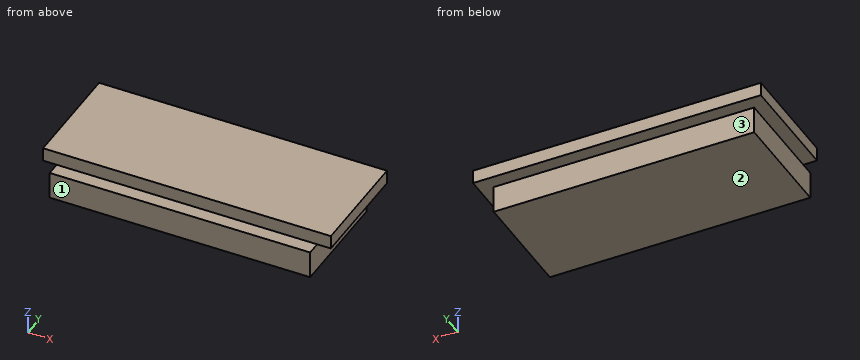
Autodesk Fusion 360 part; units mm, degrees
sketch "Sketch1" plane through (0, 0, 0) normal (0, 0, 1) x (1, 0, 0)
  line L0 (9.5, 4) -> (-9.5, 4)
  line L1 (-9.5, 4) -> (-9.5, -4)
  line L2 (-9.5, -4) -> (9.5, -4)
  line L3 (9.5, -4) -> (9.5, 4)
  line L4 (9.5, 4) -> (-9.5, -4) construction
  line L5 (-9.5, 4) -> (9.5, -4) construction
  dimension "d1" = 19
  dimension "d2" = 8
extrude "Extrude1" add sketch "Sketch1" along normal blind 2
sketch "Sketch2" plane through (0, 0, 2) normal (0, 0, 1) x (-1, 0, 0)
  line L0 (-9.5, 4) -> (-9.5, -4)
  line L1 (-9.5, -4) -> (9.5, -4)
  line L2 (9.5, -4) -> (9.5, 4)
  line L3 (9.5, 4) -> (-9.5, 4)
  line L4 (0, 4) -> (0, 3)
  line L5 (0, 3) -> (0, -5)
  line L6 (-10.5, -5) -> (10.5, -5)
  line L7 (10.5, -5) -> (10.5, 3)
  line L8 (10.5, 3) -> (-10.5, 3)
  line L9 (-10.5, 3) -> (-10.5, -5)
  line L10 (-10.5, -5) -> (10.5, 3) construction
  line L11 (10.5, -5) -> (-10.5, 3) construction
  dimension "d5" = 21
extrude "Extrude2" add sketch "Sketch2" along normal blind 1 contours L0 L1 L5 L8 | L0 L1 L5 L6 L8 L9 | L1 L2 L5 L8 | L1 L2 L5 L6 L7 L8
Verification items for the finished model (mm, model axes). Face numbers are marked on the shaded views. Coordinates: 2 decimals unless noted, no trailing zeros. Write each loop counter-clockwise with the first axis right and the second up, starting at its lowest first coordinate (ties: lowest second). Pieces come first, ordered by that corner, then holes. Notation, with made-up numbers: (53, -15.75) -> (83, -15.75) arc R21 cw to (83, 6.25) -> close; hole circle Ø9 at (-20, 5). An arc over 180 degrees is marked (long way). One line per item, written item: value. Start each with the question number.
Q1. Mould release check, pull along Y, two halves, no side actions. Record for the marked faces 1, 2 and 3: pulls with the +Y half, pulls with the -Y half, needs draft (parallel to the pull), parting line crosses it, or undercut.
Q2. Thickness scan on L1, parallel to Y at x = -3, z = 1.5; L2, parallel to X at y = -1.75, z = 0.9; L3, parallel to Y at x = 8.25, z = 2.35. Record the ranges inside material, lowest first. Write a range as from..to.
Q3. Go/stop test with flat-tipped pins: P1, Ø1, axis at x = -4.5, z = 1, coming from the +Y side; P2, Ø1, axis at y = -1, z = 0.5, coming from the -X side; P3, Ø0.5, axis at x = -1.5, y = -3.5, coming from the +Z side; P4, Ø1.5, axis at x = 6, z = 2.5, coming from the -Y side. Record where each tip stops, or that it passes through.
Q4. Cross-section at B-B on x = -3.5. Enter the section's corners in (y, z).
Q5. Cross-section at A-A on y = -2. Enter the section's corners in (x, z), and give its area (3 significant figures).
Q6. Cross-section at C-C on z = 1.4. Enter the section's corners in (x, y).
Q7. Cross-section at D-D on y = 4.75. Enter the section's corners in (x, z).
Checked values:
1. face 1: pulls with the -Y half
1. face 2: needs draft
1. face 3: pulls with the +Y half
2. L1: y = -4..4
2. L2: x = -9.5..9.5
2. L3: y = -3..5
3. P1: stops at y = 4
3. P2: stops at x = -9.5
3. P3: stops at z = 2
3. P4: stops at y = -4
4. outline: (-4, 0) -> (4, 0) -> (4, 2) -> (5, 2) -> (5, 3) -> (-3, 3) -> (-3, 2) -> (-4, 2) -> close
5. outline: (-10.5, 2) -> (-9.5, 2) -> (-9.5, 0) -> (9.5, 0) -> (9.5, 2) -> (10.5, 2) -> (10.5, 3) -> (-10.5, 3) -> close
5. area: 59.0 mm²
6. outline: (-9.5, -4) -> (9.5, -4) -> (9.5, 4) -> (-9.5, 4) -> close
7. outline: (-10.5, 2) -> (10.5, 2) -> (10.5, 3) -> (-10.5, 3) -> close
